Here's the drawing with two shaded views (mm, measured from the low corner). I have some questions. Give positions to 0.01 mm unless a question says otherwise; leave off trailing zeros. Loops run counter-clockwise (first coordinate to the right, second up) from the corner with the lowest first, then second, coordinate; pieces in that order, holes last. Notation, with made-up numbers: (-35.5, 22) -> (19.5, 22) arc R5 ccw to (19.5, 27) -> close; hole circle Ø9 at (63, -26). An arc over 180 degrees is marked (long way). Answer in a Markdown table with one row per item. Add a question column.
Item 1: If we section it at C-C (y = 1): Give the number of separate pieces and of enclosed holes in the cut face.
Item 2: For P1, Ø2.5, axis at x = 144.78, z = 7.62, coming from the -Y side; P2, Ø5.5, axis at x = 144.78, z = 144.78, coming from the +Y side (3 decimals), each with a flat end and sliding along its axis, tell me the tip position at first contact or that it passes through.
Item 3: If I drill on line 1 (Z direction, x = 65.5, y = 1); line 2 (Z direction, x = 76.2, y = 1.5); line 3 (Z direction, x = 12, y = 2.8), over which ranges is the centre line in solid material (lowest first)?
Item 4: If we section it at A-A (x = 45): Write out the boundary of the cut face in (y, z) (1 decimal), then the cut area to 3 significant figures.
Item 5: If we section it at B-B (z = 107.5): Write out the boundary of the cut face in (x, y) (1 decimal).
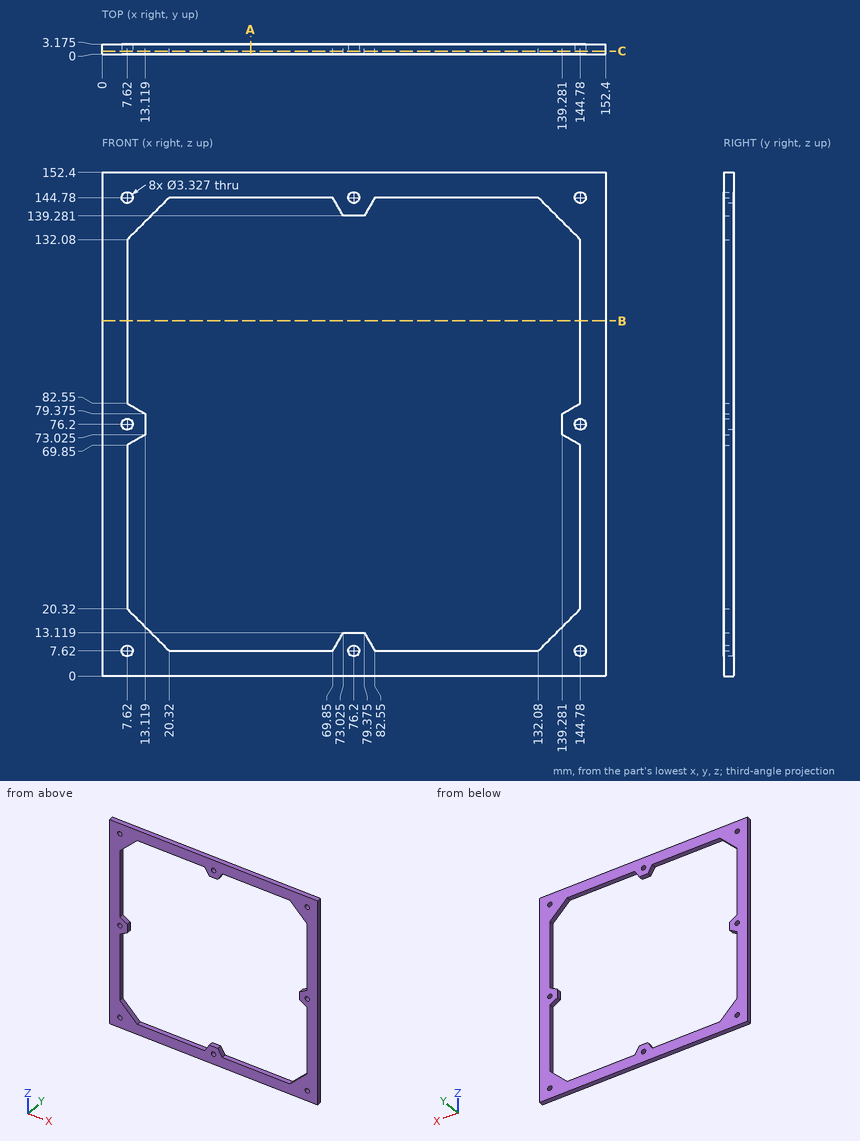
Recorded:
| question | item | result |
|---|---|---|
| 1 | separate pieces | 1 |
| 1 | enclosed holes | 9 |
| 2 | P1 | passes through |
| 2 | P2 | stops at y = 3.175 |
| 3 | line 1 | z = 0 to 7.62, 144.78 to 152.4 |
| 3 | line 2 | z = 0 to 5.96, 9.28 to 13.12, 139.28 to 143.12, 146.44 to 152.4 |
| 3 | line 3 | z = 0 to 15.94, 72.38 to 80.02, 136.46 to 152.4 |
| 4 | outline | (0, 0) -> (3.2, 0) -> (3.2, 7.6) -> (0, 7.6) -> close; (0, 144.8) -> (3.2, 144.8) -> (3.2, 152.4) -> (0, 152.4) -> close |
| 4 | area | 48.4 mm^2 |
| 5 | outline | (0, 0) -> (7.6, 0) -> (7.6, 3.2) -> (0, 3.2) -> close; (144.8, 0) -> (152.4, 0) -> (152.4, 3.2) -> (144.8, 3.2) -> close |
